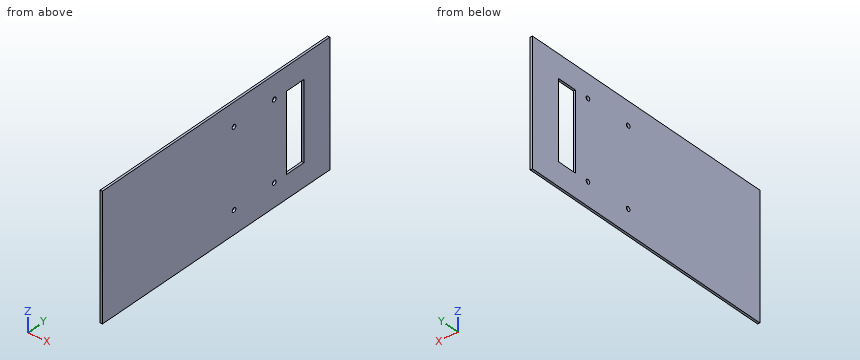
```python
from build123d import *

# Parameters (mm, degrees)
SKETCH1_W           = 174.91964
SKETCH1_H           = 381.5334
SKETCH1_R           = 3.015623361
SKETCH1_W_2         = 109.668996446
SKETCH1_H_2         = 28.739233449
BOSS_EXTRUDE1_DEPTH = 3.175


with BuildPart() as part:
    # Sketch1 → Boss-Extrude1 (new body)
    with BuildSketch(Plane(origin=(0, 0, 0), x_dir=(0, 0, -1), z_dir=(1, 0, 0))):
        Rectangle(SKETCH1_W, SKETCH1_H)
        with Locations((-54.834498223, 97.534188116)):
            Circle(SKETCH1_R, mode=Mode.SUBTRACT)
        with Locations((54.834498223, 97.534188116)):
            Circle(SKETCH1_R, mode=Mode.SUBTRACT)
        with Locations((54.834498223, 30.034188116)):
            Circle(SKETCH1_R, mode=Mode.SUBTRACT)
        with Locations((-54.834498223, 30.034188116)):
            Circle(SKETCH1_R, mode=Mode.SUBTRACT)
        with Locations((0, 132.82288111)):
            Rectangle(SKETCH1_W_2, SKETCH1_H_2, mode=Mode.SUBTRACT)
    extrude(amount=BOSS_EXTRUDE1_DEPTH)


solid = part.part
```
The model under review builds one solid part; all positions refer to its coordinate system, in mm. Give positions to 0.01 mm unless a question says otherwise; leave off trailing zeros. Loops run counter-clockwise (first coordinate to the right, second up) from the corner with the lowest first, then second, coordinate; pieces in that order, holes last. Notation, with made-up numbers: (70.5, -29) - (91.5, -29) arc R26 cw to (91.5, 7) - close; hole circle Ø8 at (11, 79). An arc over 180 degrees is marked (long way). Answer as a JSON object with one key per item and string values.
Q1. Add section B-B on y = 133.5. State the section outline as (x, z) points (1 decimal).
Worked out:
{"outline": "(0, -87.5) - (3.2, -87.5) - (3.2, -54.8) - (0, -54.8) - close; (0, 54.8) - (3.2, 54.8) - (3.2, 87.5) - (0, 87.5) - close"}
Q2. Add section A-A on z = -40.5. State the section outline as (x, y) points (1 decimal).
Worked out:
{"outline": "(0, -190.8) - (3.2, -190.8) - (3.2, 118.5) - (0, 118.5) - close; (0, 147.2) - (3.2, 147.2) - (3.2, 190.8) - (0, 190.8) - close"}
Q3. To check wall thickness, follow line 1 along Y through (x, z) = (1, -7); line 2 along Z through (x, y) = (2, 128.5). State the ranges of each line that lie inside material, in increasing order.
Worked out:
{"line 1": "y = -190.77 to 118.45, 147.19 to 190.77", "line 2": "z = -87.46 to -54.83, 54.83 to 87.46"}
Q4. Add section C-C on x = 1.2. State the section outline as (y, z) points.
Worked out:
{"outline": "(-190.77, -87.46) - (190.77, -87.46) - (190.77, 87.46) - (-190.77, 87.46) - close; hole circle Ø6.03 at (30.03, -54.83); hole circle Ø6.03 at (30.03, 54.83); hole circle Ø6.03 at (97.53, -54.83); hole circle Ø6.03 at (97.53, 54.83); hole (118.45, -54.83) - (147.19, -54.83) - (147.19, 54.83) - (118.45, 54.83) - close"}
